from build123d import *

# Parameters (mm, degrees)
F0_W     = 61
F0_H     = 146
F0_W_2   = 58
F0_H_2   = 143
F0_W_3   = 55
F0_H_3   = 140
F1_DEPTH = 2
F2_DEPTH = 28
F3_DEPTH = 30


with BuildPart() as f1:
    # F0 (on Top) → F1 (new body)
    with BuildSketch(Plane.XY):
        Rectangle(F0_W, F0_H)
        Rectangle(F0_W_2, F0_H_2, mode=Mode.SUBTRACT)
        Rectangle(F0_W_2, F0_H_2)
        Rectangle(F0_W_3, F0_H_3, mode=Mode.SUBTRACT)
        Rectangle(F0_W_3, F0_H_3)
    extrude(amount=-F1_DEPTH)

    # F0 (on Top) → F2 (join)
    with BuildSketch(Plane.XY):
        Rectangle(F0_W, F0_H)
        Rectangle(F0_W_2, F0_H_2, mode=Mode.SUBTRACT)
        Rectangle(F0_W_2, F0_H_2)
        Rectangle(F0_W_3, F0_H_3, mode=Mode.SUBTRACT)
    extrude(amount=-F2_DEPTH)

    # F0 (on Top) → F3 (join)
    with BuildSketch(Plane.XY):
        Rectangle(F0_W, F0_H)
        Rectangle(F0_W_2, F0_H_2, mode=Mode.SUBTRACT)
    extrude(amount=-F3_DEPTH)


solid = f1.part
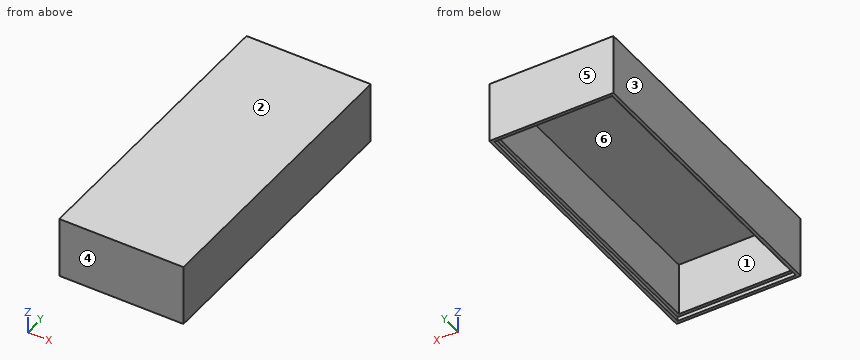
The model under review builds one solid part; all positions refer to its coordinate system, in mm. Face numbers are marked on the shaded views. A direction names the side the tool comes from. Round coordinates to 2 decimals unless told otherwise and drop trailing zeros. Loops run counter-clockwise (first coordinate to the right, second up) from the corner with the lowest first, then second, coordinate; pieces in that order, holes last. Notation, with made-up numbers: (22, 36) -> (51, 36) arc R12 cw to (51, 51) -> close; hole circle Ø8 at (64.5, 30.25). An arc over 180 degrees is marked (long way). Return JSON: item names as keys, results as strings.
(1) Add section C-C on y = 25.5. Write out the cut boundary in (x, z).
Solved:
{"outline": "(-30.5, -30) -> (-29, -30) -> (-29, -28) -> (-27.5, -28) -> (-27.5, -2) -> (27.5, -2) -> (27.5, -28) -> (29, -28) -> (29, -30) -> (30.5, -30) -> (30.5, 0) -> (-30.5, 0) -> close"}
(2) For pin 1 (3 mm diameter, centred on x = -0.5, y = -55, fed in from -Z), flat-tipped, find the tip position at first contact; note if it passes through.
Solved:
{"pin 1": "z = -2"}
(3) The part is to be moulded in two halves that separate along Y. For the marked faces 3, 4, 5 and 6, say which applies: released by +Y, released by -Y, zero draft, split by the parting line, or undercut.
Solved:
{"face 3": "zero draft", "face 4": "released by -Y", "face 5": "released by +Y", "face 6": "undercut"}
(4) For the marked faces 1 and 2, list the 3-axis set-ups (+Z, -Z, +X, -X, +Y, -Y) from which the entire face can be reached by the end or side of a thin tool; tool diameter is ignored.
Solved:
{"face 1": "-Z", "face 2": "+Z, +X, -X, +Y, -Y"}
(5) Add section A-A on z = -15.25. Write out the cut boundary in (x, y), plus the area to 3 significant figures.
Solved:
{"outline": "(-30.5, -73) -> (30.5, -73) -> (30.5, 73) -> (-30.5, 73) -> close; hole (-27.5, -70) -> (27.5, -70) -> (27.5, 70) -> (-27.5, 70) -> close", "area": "1,210 mm2"}
(6) Add section B-B on x = -10. Write out the cut boundary in (y, z).
Solved:
{"outline": "(-73, -30) -> (-71.5, -30) -> (-71.5, -28) -> (-70, -28) -> (-70, -2) -> (70, -2) -> (70, -28) -> (71.5, -28) -> (71.5, -30) -> (73, -30) -> (73, 0) -> (-73, 0) -> close"}
(7) For line 1 (X direction, y = -56, z = -24.5); line 2 (Y direction, x = 25.5, z = -7.25); line 3 (Z direction, x = -12, y = 49), list the stretches that pass through material, from the lowest coordinate up.
Solved:
{"line 1": "-30.5 to -27.5, 27.5 to 30.5", "line 2": "-73 to -70, 70 to 73", "line 3": "-2 to 0"}
